The listing builds one solid part. Answer for the finished solid, in the listing's coordinates (mm). Coordinates: 2 decimals unless noted, no trailing zeros. Write each loop counter-clockwise with the first axis right and the second up, starting at its lowest first coordinate (ties: lowest second). Pieces come first, ordered by that corner, then holes.
from build123d import *

# Parameters (mm, degrees)
SKETCH1_W           = 762
SKETCH1_H           = 12.7
BOSS_EXTRUDE1_DEPTH = 609.6
SKETCH2_W           = 12.7
SKETCH2_H           = 609.6
BOSS_EXTRUDE2_DEPTH = 76.2
SKETCH3_OUTSIDE_W   = 1136.21
SKETCH3_OUTSIDE_H   = 831.41
CUT_EXTRUDE1_DEPTH  = 12.7
SKETCH6_W           = 56.167651581
SKETCH6_H           = 12.7
SKETCH6_W_2         = 683.835303162
CUT_EXTRUDE2_DEPTH  = 12.7
SKETCH7_W           = 12.7
SKETCH7_H           = 88.9
CUT_EXTRUDE3_DEPTH  = 12.7
BOSS_EXTRUDE3_START = -101.6
SKETCH8_W           = 732.670606326
SKETCH8_H           = 12.7
BOSS_EXTRUDE3_DEPTH = 101.6
BOSS_EXTRUDE4_START = -12.7
SKETCH9_W           = 68.867651581
SKETCH9_H           = 12.7
BOSS_EXTRUDE4_DEPTH = 12.7


with BuildPart() as part:
    # Sketch1 → Boss-Extrude1 (new body)
    with BuildSketch(Plane(origin=(0, 0, 0), x_dir=(1, 0, 0), z_dir=(0, 1, 0))):
        with Locations((0, -653.561357684)):
            Rectangle(SKETCH1_W, SKETCH1_H)
    extrude(amount=BOSS_EXTRUDE1_DEPTH)

    # Sketch2 → Boss-Extrude2 (add)
    with BuildSketch(Plane(origin=(381, 0, 0), x_dir=(0, 0, -1), z_dir=(1, 0, 0))):
        with Locations((-653.561357684, 304.8)):
            Rectangle(SKETCH2_W, SKETCH2_H)
    boss_extrude2 = extrude(amount=BOSS_EXTRUDE2_DEPTH)

    # Mirror1: Boss-Extrude2 across plane
    add(boss_extrude2.mirror(Plane(origin=(0, 0, 0), x_dir=(0, 0, 1), z_dir=(1, 0, 0))))

    # Sketch3 outside → Cut-Extrude1 (cut)
    with BuildSketch(Plane.XY.offset(659.911357684)):
        with Locations((0, 304.8)):
            Rectangle(SKETCH3_OUTSIDE_W, SKETCH3_OUTSIDE_H)
        Polygon((366.335303163, 609.6), (-366.335303163, 609.6), (-366.335303163, 533.4), (-388.332348419, 533.4), (-388.332348419, 609.6), (-457.2, 609.6), (-457.2, 457.2), (-366.335303163, 457.2), (-366.335303163, 304.8), (-388.332348419, 304.8), (-388.332348419, 381), (-457.2, 381), (-457.2, 228.6), (-366.335303163, 228.6), (-366.335303163, 76.2), (-388.332348419, 76.2), (-388.332348419, 152.4), (-457.2, 152.4), (-457.2, 0), (457.2, 0), (457.2, 152.4), (388.332348419, 152.4), (388.332348419, 76.2), (366.335303163, 76.2), (366.335303163, 228.6), (457.2, 228.6), (457.2, 381), (388.332348419, 381), (388.332348419, 304.8), (366.335303163, 304.8), (366.335303163, 457.2), (457.2, 457.2), (457.2, 609.6), (388.332348419, 609.6), (388.332348419, 533.4), (366.335303163, 533.4), align=None, mode=Mode.SUBTRACT)
    extrude(amount=-CUT_EXTRUDE1_DEPTH, mode=Mode.SUBTRACT)

    # Sketch6 → Cut-Extrude2 (cut)
    with BuildSketch(Plane(origin=(0, 609.6, 0), x_dir=(1, 0, 0), z_dir=(0, 1, 0))):
        with Locations((-416.41617421, -653.561357684)):
            Rectangle(SKETCH6_W, SKETCH6_H)
        with Locations((0, -653.561357684)):
            Rectangle(SKETCH6_W_2, SKETCH6_H)
        with Locations((416.41617421, -653.561357684)):
            Rectangle(SKETCH6_W, SKETCH6_H)
    cut_extrude2 = extrude(amount=-CUT_EXTRUDE2_DEPTH, mode=Mode.SUBTRACT)

    # Sketch7 → Cut-Extrude3 (cut)
    with BuildSketch(Plane.XY.offset(659.911357684)):
        with Locations((154.820606325, 552.45)):
            Rectangle(SKETCH7_W, SKETCH7_H)
        with Locations((-154.820606325, 552.45)):
            Rectangle(SKETCH7_W, SKETCH7_H)
    cut_extrude3 = extrude(amount=-CUT_EXTRUDE3_DEPTH, mode=Mode.SUBTRACT)

    # Mirror2: Cut-Extrude2, Cut-Extrude3 across plane
    add(cut_extrude2.mirror(Plane(origin=(0, 304.8, 0), x_dir=(0, 0, 1), z_dir=(0, -1, 0))), mode=Mode.SUBTRACT)
    add(cut_extrude3.mirror(Plane(origin=(0, 304.8, 0), x_dir=(0, 0, 1), z_dir=(0, -1, 0))), mode=Mode.SUBTRACT)

    # Sketch8 → Boss-Extrude3 (add)
    with BuildSketch(Plane(origin=(0, 609.6, 0), x_dir=(1, 0, 0), z_dir=(0, 1, 0)).offset(BOSS_EXTRUDE3_START)):
        with Locations((0, -653.561357684)):
            Rectangle(SKETCH8_W, SKETCH8_H)
    extrude(amount=BOSS_EXTRUDE3_DEPTH)

    # Sketch9 → Boss-Extrude4 (add)
    with BuildSketch(Plane(origin=(0, 609.6, 0), x_dir=(1, 0, 0), z_dir=(0, 1, 0)).offset(BOSS_EXTRUDE4_START)):
        with Locations((422.76617421, -653.561357684)):
            Rectangle(SKETCH9_W, SKETCH9_H)
        with Locations((-422.76617421, -653.561357684)):
            Rectangle(SKETCH9_W, SKETCH9_H)
    extrude(amount=BOSS_EXTRUDE4_DEPTH)


solid = part.part
Q1. The part is cut by section B-B, the plane x = 213.5. Write down the section's boundary in (y, z).
Answers below:
outline: (12.7, 647.21) - (609.6, 647.21) - (609.6, 659.91) - (12.7, 659.91) - close
Q2. The part is cut by section C-C, the plane y = 218.5. Write down the section's boundary in (x, z), then the cut area to 3 significant figures.
Answers below:
outline: (-366.34, 647.21) - (366.34, 647.21) - (366.34, 659.91) - (-366.34, 659.91) - close
area: 9,300 mm2
Q3. Given pin 1 (1 mm diameter, centred on x = 285.5, z = 657, fed in from -Y); pin 2 (1 mm diameter, centred on y = 396, z = 648.5, fed in from +X); pin 3 (4 mm diameter, centred on x = -153.5, z = 656, fed in from -Y), each flat-ended and moving along its own axis, determine where each tip first touches the part or whether it passes through.
Answers below:
pin 1: stops at y = 12.7
pin 2: stops at x = 366.34
pin 3: stops at y = 101.6
Q4. The part is cut by section A-A, the plane y = 543.5. Write down the section's boundary in (x, z).
Answers below:
outline: (-457.2, 647.21) - (-388.33, 647.21) - (-388.33, 659.91) - (-457.2, 659.91) - close; (-366.34, 647.21) - (366.34, 647.21) - (366.34, 659.91) - (-366.34, 659.91) - close; (388.33, 647.21) - (457.2, 647.21) - (457.2, 659.91) - (388.33, 659.91) - close
Q5. Find the intervals of material crossed by probe 1 along X at (y, z) = (32.5, 654); probe 2 along X at (y, z) = (329, 651.5); probe 3 along X at (y, z) = (93.5, 653.5), in increasing order.
Answers below:
probe 1: x = -457.2 to -161.17, -148.47 to 148.47, 161.17 to 457.2
probe 2: x = -457.2 to -388.33, -366.34 to 366.34, 388.33 to 457.2
probe 3: x = -457.2 to -388.33, -366.34 to -161.17, -148.47 to 148.47, 161.17 to 366.34, 388.33 to 457.2
